The listing builds one solid part. Answer for the finished solid, in the listing's coordinates (mm). A direction names the side the tool comes from. Round coordinates to 2 decimals unless told otherwise and drop trailing zeros. Write each loop counter-clockwise with the first axis right and the second up, starting at its lowest first coordinate (ties: lowest second). Pieces come first, ordered by that corner, then holes. Notation, with made-up numbers: (14.5, 16) - (62.5, 16) arc R26 ccw to (62.5, 47) - close; hole circle Ø1 at (49.25, 36). An arc over 180 degrees is marked (long way). Answer in a Markdown table with one row per item.
from build123d import *

# Parameters (mm, degrees)
F0_W     = 152.4
F0_H     = 50
F1_DEPTH = 3
F2_W     = 5.4
F2_H     = 13
F3_DEPTH = 3.001


with BuildPart() as f1:
    # F0 (on Top) → F1 (new body)
    with BuildSketch(Plane.XY):
        Rectangle(F0_W, F0_H)
    extrude(amount=F1_DEPTH)

    # F2 (on face) → F3 (cut, through all)
    with BuildSketch(Plane.XY.offset(3)):
        with Locations((-71.4075, 0)):
            Rectangle(F2_W, F2_H)
        with Locations((-61.8225, 0)):
            Rectangle(F2_W, F2_H)
        with Locations((-52.2375, 0)):
            Rectangle(F2_W, F2_H)
        with Locations((-42.6525, 0)):
            Rectangle(F2_W, F2_H)
        with Locations((-33.0675, 0)):
            Rectangle(F2_W, F2_H)
        with Locations((-23.4825, 0)):
            Rectangle(F2_W, F2_H)
        with Locations((-13.8975, 0)):
            Rectangle(F2_W, F2_H)
        with Locations((-4.3125, 0)):
            Rectangle(F2_W, F2_H)
        with Locations((5.2725, 0)):
            Rectangle(F2_W, F2_H)
        with Locations((14.8575, 0)):
            Rectangle(F2_W, F2_H)
    extrude(amount=-F3_DEPTH, mode=Mode.SUBTRACT)


solid = f1.part
(1) Section A-A (x = -51.5) is taken. Give the vertices of the cut face in (y, z), and give its area (3 significant figures).
Checked values:
| item | result |
|---|---|
| outline | (-25, 0) - (-6.5, 0) - (-6.5, 3) - (-25, 3) - close; (6.5, 0) - (25, 0) - (25, 3) - (6.5, 3) - close |
| area | 111 mm2 |
(2) Section B-B (y = 1) is taken. State how many separate pieces and enclosed holes the cut face has, and give its area (3 significant figures).
Checked values:
| item | result |
|---|---|
| separate pieces | 11 |
| enclosed holes | 0 |
| area | 295 mm2 |
(3) Find the intervals of material crossed by line 1 (Y direction, x = -62, z = 1.1), in increasing order.
Checked values:
| item | result |
|---|---|
| line 1 | y = -25 to -6.5, 6.5 to 25 |
(4) For faces 3 (the flat face through (-1, 25, 1)), 4 (the flat face through (-1.612, 0, 2)), determine the directions among +Z, -Z, +X, -X, +Y, -Y from which every point of the face is accessible in a straight line to the end or side of a thin tool.
Checked values:
| item | result |
|---|---|
| face 3 | +Z, -Z, +X, -X, +Y |
| face 4 | +Z, -Z |
(5) For a pull along X with two mould halves and no side action, classify faces 1 (the flat face through (-1, -25, 1)), 2 (the flat face through (12.157, 0, 2)) as pulls with the +X half, pulls with the -X half, needs draft (parallel to the pull), parting line crosses it, or undercut.
Checked values:
| item | result |
|---|---|
| face 1 | needs draft |
| face 2 | undercut |
